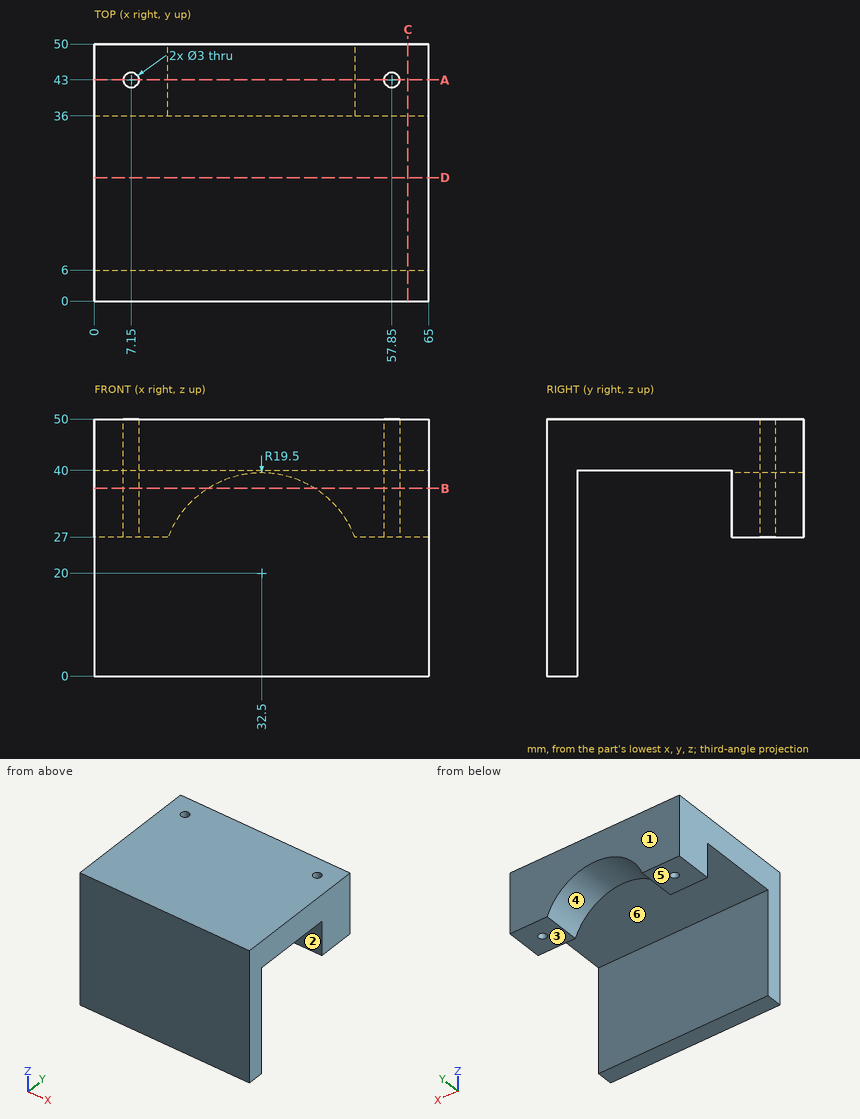
Input: dimensioned drawing with shaded views. Units: mm. Origin: part minimum x, y, z. A direction names the side the tool comes from. Coordinates: 2 decimals unless noted, no trailing zeros. Write each loop counter-clockwise with the first axis right and the second up, starting at its lowest first coordinate (ties: lowest second). Pieces come first, ordered by that corner, then holes. Notation, with made-up numbers: M 42.5,33.5 L 75.5,33.5 A31 cw 75.5,58.5 Z; hole C 69.5,-1 d11. An arc over 180 degrees is marked long. Answer as CSV lines item,"result". Start each with the question number.
Q1. Cut plane C-C on x = 61. Return the cut outline in (y, z), then the cut area to 3 significant figures.
Q2. Cut plane B-B on z = 36.5. Return the cut outline in (x, y).
Q3. Reachability of the marked faces 4, 5 and 6 from +Z, -Z, +X, -X, +Y, -Y: full face, straight path, thin tool, end or side. Return the list, or none.
Q4. Cut plane D-D on y = 24. Return the cut outline in (x, z).
Q5. Cut plane A-A on y = 43. Return the cut outline in (x, z).
Q6. Mould query, pull axis Y, two halves, no side actions, for the marked faces 1, 2 and 3. Classes: released by +Y, released by -Y, zero draft, split by the parting line, or undercut.
Q7. Line query: line 1 (Y direction, x = 54, z = 32); line 2 (Z direction, x = 12.5, y = 19.5); line 3 (Y direction, x = 42.5, z = 19.5). Output: solid intervals per line, ascending. Write a range as from..to.
Q8. Pin query (flat end, axial travel): P1, Ø11, axis at x = 58.5, y = 43.5, coming from the -Z side; P2, Ø3, axis at x = 31, z = 15, coming from the +Y side; P3, Ø2.5, axis at x = 7.15, y = 43, coming from the +Z side; P4, Ø6, axis at x = 38.5, z = 35, coming from the -Y side. Return the tip coordinate at first contact, or that it passes through.
Findings below:
1,outline,"M 0,0 L 6,0 L 6,40 L 36,40 L 36,27 L 50,27 L 50,50 L 0,50 Z"
1,area,"922 mm2"
2,outline,"M 0,0 L 65,0 L 65,6 L 0,6 Z; M 0,36 L 22.11,36 L 22.11,50 L 0,50 Z; M 42.89,36 L 65,36 L 65,50 L 42.89,50 Z; hole C 7.15,43 d3; hole C 57.85,43 d3"
3,face 4,"-Z, +Y"
3,face 5,"-Z, +X, -X, +Y"
3,face 6,"-Z, +X, -X"
4,outline,"M 0,40 L 65,40 L 65,50 L 0,50 Z"
5,outline,"M 0,27 L 5.65,27 L 5.65,50 L 0,50 Z; M 8.65,27 L 14.3,27 A19.5 cw 50.7,27 L 56.35,27 L 56.35,50 L 8.65,50 Z; M 59.35,27 L 65,27 L 65,50 L 59.35,50 Z"
6,face 1,"released by +Y"
6,face 2,"undercut"
6,face 3,"zero draft"
7,line 1,"y = 0..6, 36..50"
7,line 2,"z = 40..50"
7,line 3,"y = 0..6"
8,P1,"stops at z = 27"
8,P2,"stops at y = 6"
8,P3,"passes through"
8,P4,"stops at y = 0"
